from build123d import *

# Parameters (mm, degrees)
BOSS_EXTRUDE1_DEPTH = 18


with BuildPart() as part:
    # Sketch1 → Boss-Extrude1 (new body)
    with BuildSketch(Plane.XY):
        with BuildLine():
            Line((-7.163105934, -7.293646663), (-6.547062338, -6.677603067))
            Line((-6.547062338, -6.677603067), (-6.612332703, -6.612332703))
            Line((-6.612332703, -6.612332703), (-7.563291756, -5.661373649))
            ThreePointArc((-7.563291756, -5.661373649), (-8.288491154, -4.742354928), (-8.78011552, -3.679897843))
            ThreePointArc((-8.78011552, -3.679897843), (-9.870465754, -2.18361858), (-11.631530122, -1.612332703))
            Line((-11.631530122, -1.612332703), (-14.432396648, -1.612332703))
            ThreePointArc((-14.432396648, -1.612332703), (-16.193461017, -2.18361858), (-17.28381125, -3.679897843))
            ThreePointArc((-17.28381125, -3.679897843), (-17.775435616, -4.742354928), (-18.500635014, -5.661373649))
            Line((-18.500635014, -5.661373649), (-19.451594068, -6.612332703))
            Line((-19.451594068, -6.612332703), (-19.524780345, -6.680666225))
            Line((-19.524780345, -6.680666225), (-18.670477775, -7.534870352))
            add(Edge.make_bspline(
                [(-18.670477775, -7.534870352), (-18.125131144, -8.012979969), (-17.277228248, -8.540037204), (-16.066456083, -8.958058574), (-14.806247878, -9.200473351), (-13.120861063, -9.255335571), (-11.668367706, -9.128182371), (-10.874120868, -9.043245859), (-10.794454533, -9.034648972)],
                knots=[0, 0, 0, 0, 0.231047832, 0.35138283, 0.481745746, 0.716877708, 0.971604001, 1, 1, 1, 1], degree=3, weights=[1, 1, 1, 1, 1, 1, 1, 1, 1]))
            add(Edge.make_bspline(
                [(-7.163105934, -7.293646663), (-7.528267353, -7.658808082), (-7.948111458, -7.955995317), (-8.369394277, -8.254200947), (-8.833411811, -8.476523795), (-9.296011092, -8.69816712), (-9.792074347, -8.839471582), (-10.28381467, -8.979544649), (-10.794454533, -9.034648972)],
                knots=[0, 0, 0, 0.25, 0.25, 0.5, 0.5, 0.75, 0.75, 1, 1, 1], degree=2))
        make_face()
    extrude(amount=-BOSS_EXTRUDE1_DEPTH)


solid = part.part
Input: part model. Units: mm. Frame: model coordinates. Coordinates: 2 decimals unless noted, no trailing zeros. Loops run counter-clockwise (first coordinate to the right, second up) from the corner with the lowest first, then second, coordinate; pieces in that order, holes last. Notation, with made-up numbers: (-12, 48.25) - (39, 48.25) arc R22 ccw to (39, 54.25) - close; hole circle Ø10 at (80, -6). An arc over 180 degrees is marked (long way). Answer in a Markdown table with one row per item. Add a question column.
Item 1: Line query: line 1 along Y through (x, z) = (-13.25, -8); line 2 along Y through (x, z) = (-8.5, -7); line 3 along X through (y, z) = (-3.25, -14.25). Output: solid intervals per line, ascending. Write a range as [from, to].
Item 2: Section query B-B on y = -6. Return the cut outline in (x, z).
Item 3: Contact query for flat-ended pins moving along their axis: P1, Ø3, axis at y = -8.5, z = -11.5, coming from the +X side; P2, Ø1.5, axis at x = -8, z = -8.5, coming from the -Y side. Output: stop coordinate, or through.
Item 4: Section query A-A on y = -5. Return the cut outline in (x, z).
Recorded:
| question | item | result |
|---|---|---|
| 1 | line 1 | [-9.22, -1.61] |
| 1 | line 2 | [-8.3, -4.36] |
| 1 | line 3 | [-17.11, -8.96] |
| 2 | outline | (-18.84, -18) - (-7.22, -18) - (-7.22, 0) - (-18.84, 0) - close |
| 3 | P1 | x = -6.87 |
| 3 | P2 | y = -8.44 |
| 4 | outline | (-17.94, -18) - (-8.12, -18) - (-8.12, 0) - (-17.94, 0) - close |
